from build123d import *

# Parameters (mm, degrees)
F0_R     = 3
F1_DEPTH = 22
F2_R     = 1.931371
F3_R     = 1.5
F4_DEPTH = 2


with BuildPart() as f1:
    # F0 (on Top) → F1 (new body)
    with BuildSketch(Plane.XY):
        Circle(F0_R)
    extrude(amount=F1_DEPTH)

    # F2
    f2_edges = [f1.edges().sort_by_distance(p)[0] for p in [
        (-3, 0, 22),
    ]]
    fillet(f2_edges, radius=F2_R)

    # F3 (on face) → F4 (join)
    with BuildSketch(Plane(origin=(0, 0, 0), x_dir=(1, 0, 0), z_dir=(0, 0, -1))):
        Circle(F3_R)
    extrude(amount=F4_DEPTH)


solid = f1.part
Build history of the part. All positions in model axes, mm. A direction names the side the tool comes from. Round coordinates to 2 decimals unless told otherwise and drop trailing zeros. Write each loop counter-clockwise with the first axis right and the second up, starting at its lowest first coordinate (ties: lowest second). Pieces come first, ordered by that corner, then holes. Notation, with made-up numbers: (32, -15.5) - (45, -15.5) arc R16 ccw to (45, 15.5) - close; hole circle Ø5 at (38, 8.5). An arc over 180 degrees is marked (long way). One line per question, with ' | ' between items.
1. Drop flat-ended pins along their axis: pin 1 Ø1.5 at (x, z) = (-2.5, 19) entering from -Y; pin 2 Ø1 at (x, y) = (-1, -1) entering from +Z; pin 3 Ø1.5 at (x, y) = (2, -2) entering from -Z; pin 4 Ø1.5 at (y, z) = (1.5, 8.5) entering from -X. Give the stop position or say it passes through.
Results are:
pin 1: y = -2.44 | pin 2: z = 22 | pin 3: z = 0 | pin 4: x = -2.9
2. Drill centre lines: line 1 along X through (y, z) = (1.55, 4.5); line 2 along Y through (x, z) = (1.8, 15.75); line 3 along Z through (x, y) = (-1.35, 0.45). Where is each one in solid material? Low to high. Write a range as from..to.
Results are:
line 1: -2.57..2.57 | line 2: -2.4..2.4 | line 3: -2..21.97
3. Tool access for faces 1 (the face through (1.3, -1.3, 0)), 2 (the face through (0, 0, -2)): list every direction of +Z, -Z, +X, -X, +Y, -Y with a clear straight run to the whole face (end or side of a thin tool).
Results are:
face 1: -Z | face 2: -Z, +X, -X, +Y, -Y
4. Band-saw the part on A-A, the plane z = 16.5. Write the cut outline in (x, y).
Results are:
outline: circle Ø6 at (0, 0)
